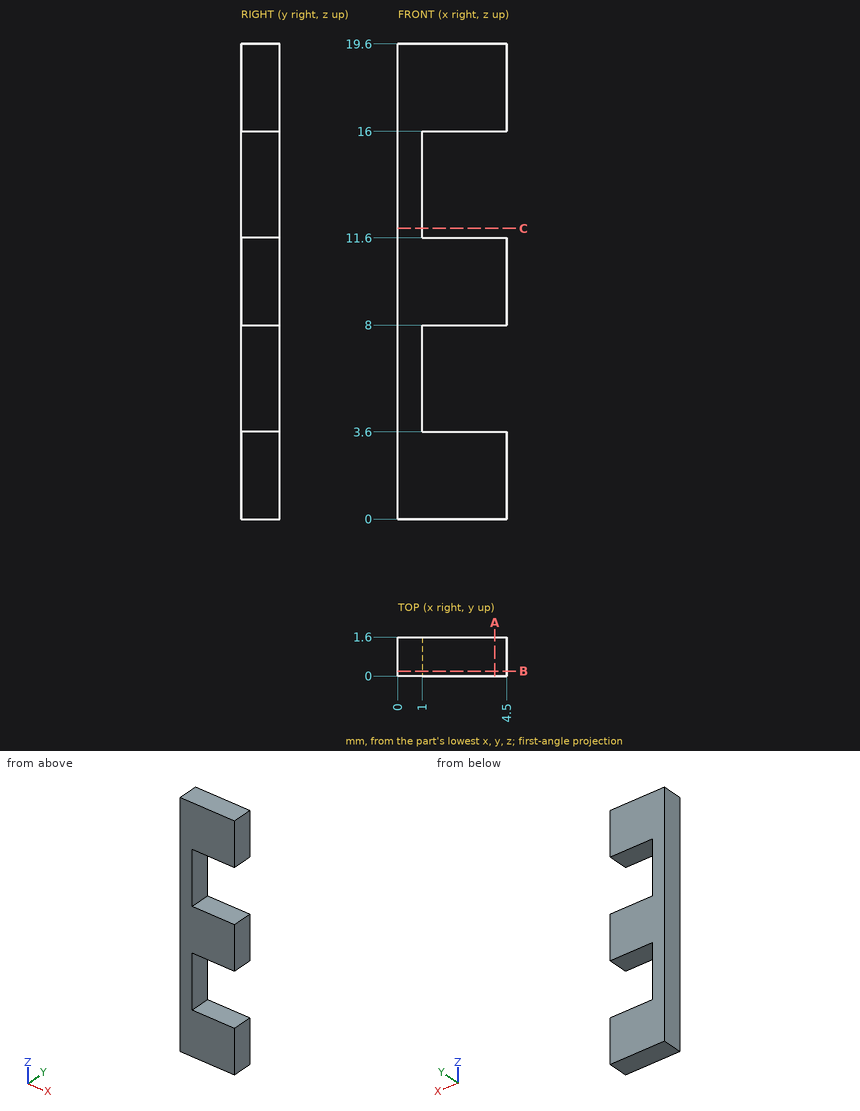
Here's the drawing with two shaded views (mm, measured from the low corner). I have some questions. Give positions to 0.01 mm unless a question says otherwise; leave off trailing zeros. Order: outer loops, then holes, each group sorted by start corner. A loop starts at its lowest first (then second) coordinate and runs counter-clockwise, first axis right, second up. Notation, with made-up numbers: (-39, 3) -> (4, 3) arc R15 cw to (4, 7) -> close; hole circle Ø11 at (39.5, -37). An arc over 180 degrees is marked (long way). Use a Markdown table: item, result. Add a question column.
Item 1: Imagine slicing it at B-B on y = 0.2. Please give me the cut outline in (x, z).
Item 2: Imagine slicing it at A-A on x = 4. Please give me the cut outline in (y, z).
Item 3: I need wall thicknesses on line 1 (Z direction, x = 3.3, y = 1.25); line 2 (X direction, y = 0.25, z = 13.75). Which ranges of each line are inside material? Lowest first, please.
Item 4: Will these pins go through, and if not, where does the flat tip stop? pin 1 (0.8 mm diameter, centred on y = 0.5, z = 4.5, fed in from +X); pin 2 (1.5 mm diameter, centred on x = 2, z = 4.5, fed in from -Y).
Item 5: Imagine slicing it at C-C on z = 12. Please give me the cut outline in (x, y), plus the area to 3 significant figures.
Data:
| question | item | result |
|---|---|---|
| 1 | outline | (0, 0) -> (4.5, 0) -> (4.5, 3.6) -> (1, 3.6) -> (1, 8) -> (4.5, 8) -> (4.5, 11.6) -> (1, 11.6) -> (1, 16) -> (4.5, 16) -> (4.5, 19.6) -> (0, 19.6) -> close |
| 2 | outline | (0, 0) -> (1.6, 0) -> (1.6, 3.6) -> (0, 3.6) -> close; (0, 8) -> (1.6, 8) -> (1.6, 11.6) -> (0, 11.6) -> close; (0, 16) -> (1.6, 16) -> (1.6, 19.6) -> (0, 19.6) -> close |
| 3 | line 1 | z = 0 to 3.6, 8 to 11.6, 16 to 19.6 |
| 3 | line 2 | x = 0 to 1 |
| 4 | pin 1 | stops at x = 1 |
| 4 | pin 2 | passes through |
| 5 | outline | (0, 0) -> (1, 0) -> (1, 1.6) -> (0, 1.6) -> close |
| 5 | area | 1.60 mm² |
